Here's the drawing with two shaded views (mm, measured from the low corner). I have some questions. A direction names the side the tool comes from. Coordinates: 2 decimals unless noted, no trailing zeros. Write each loop counter-clockwise with the first axis right and the second up, starting at its lowest first coordinate (ties: lowest second). Pieces come first, ordered by that corner, then holes.
Item 1: If we section it at A-A (x = 15.5): Please give me the cut outline in (y, z).
Item 2: If we section it at C-C (x = 10): Please give me the cut outline in (y, z).
Item 3: If we section it at B-B (y = 17.5): Please give me the cut outline in (x, z).
Item 4: I'm going to push flat-ended pins straight in: pin 1 Ø8 at (x, y) = (6, 35.5) entering from -Z; pin 2 Ø3 at (y, z) = (13.5, 4.5) entering from -X; pin 3 Ø4 at (x, y) = (11, 3.5) entering from +Z. Where does each tip first touch, or does it pass through?
Item 5: If we section it at D-D (z = 36): Please give me the cut outline in (x, y).
Item 6: For the marked faces 1, 2 and 3, which set-ups out of +Z, -Z, +X, -X, +Y, -Y let a thin tool reach every point of the face, with its end or its side?
Item 7: If I drill on line 1 (Y direction, x = 2.5, z = 9); line 2 (Z direction, x = 14, y = 27.5); line 3 (Z direction, x = 12.75, y = 2), over which ranges is the centre line in solid material (lowest first)?
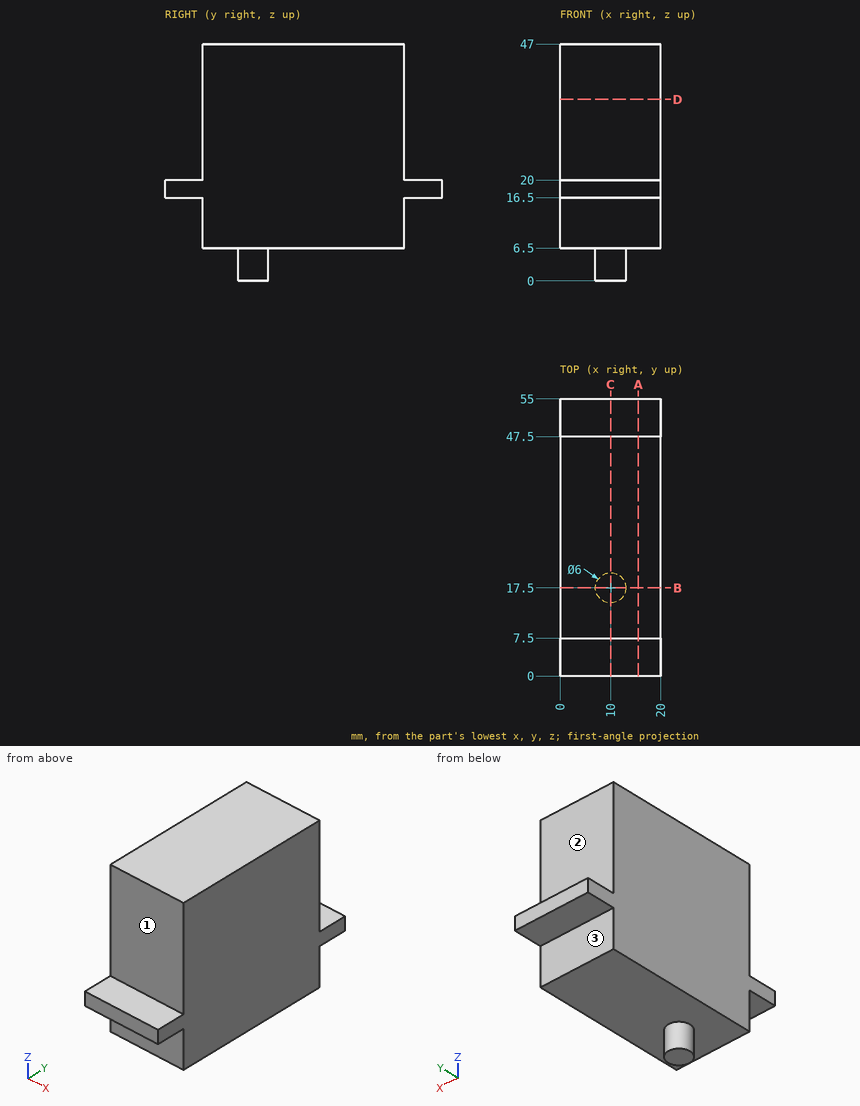
Answer list:
1. outline: (0, 16.5) - (7.5, 16.5) - (7.5, 6.5) - (47.5, 6.5) - (47.5, 16.5) - (55, 16.5) - (55, 20) - (47.5, 20) - (47.5, 47) - (7.5, 47) - (7.5, 20) - (0, 20) - close
2. outline: (0, 16.5) - (7.5, 16.5) - (7.5, 6.5) - (14.5, 6.5) - (14.5, 0) - (20.5, 0) - (20.5, 6.5) - (47.5, 6.5) - (47.5, 16.5) - (55, 16.5) - (55, 20) - (47.5, 20) - (47.5, 47) - (7.5, 47) - (7.5, 20) - (0, 20) - close
3. outline: (0, 6.5) - (7, 6.5) - (7, 0) - (13, 0) - (13, 6.5) - (20, 6.5) - (20, 47) - (0, 47) - close
4. pin 1: stops at z = 6.5
4. pin 2: stops at x = 8.34
4. pin 3: stops at z = 20
5. outline: (0, 7.5) - (20, 7.5) - (20, 47.5) - (0, 47.5) - close
6. face 1: +Z, +X, -X, -Y
6. face 2: +Z, +X, -X, +Y
6. face 3: -Z, +X, -X, +Y
7. line 1: y = 7.5 to 47.5
7. line 2: z = 6.5 to 47
7. line 3: z = 16.5 to 20
